The listing builds one solid part. Answer for the finished solid, in the listing's coordinates (mm). Face numbers are marked on the shaded views. A direction names the side the tool comes from. Round coordinates to 2 decimals unless told otherwise and drop trailing zeros. Write each loop counter-clockwise with the first axis right and the second up, starting at its lowest first coordinate (ties: lowest second). Pieces come first, ordered by that corner, then holes. Notation, with made-up numbers: (30, 49) - (85, 49) arc R13 ccw to (85, 54) - close; hole circle Ø11 at (51, -13.75). An arc over 180 degrees is marked (long way). Use a Markdown table: item, result. Add a question column.
1) A tool of negligible diameter and unlimited length cuts with its end or side. For the marked faces 5, 6, 7 and 8, from which of +Z, -Z, +X, -X, +Y, -Y can it reach the whole face along a straight path? Write none if from no direction.
2) A cutting plane is placed at D-D (z = 20.5). Give the vertices of the cut face in (x, y).
3) A cutting plane is placed at B-B (z = 4.5). Give the vertices of the cut face in (x, y), then the cut area to 3 significant figures.
4) Determine the mould class of the marked faces 1, 2, 3 and 4 for opening direction Z: +Z half, -Z half, draft (parallel to the pull), parting line (faces both ways), or undercut.
5) Each of these flat-tipped pins is pushed along its axis until it touches: P1, Ø5, axis at x = 30, z = -11.5, coming from the +Y side; P2, Ø2, axis at x = 35, y = 9, coming from the +Z side; P3, Ø3.5, axis at x = -7, z = 21, coming from the +Y side; P4, Ø5, axis at x = 33, y = 8.5, coming from the -Z side. Where does it stop, or does it pass through?
6) A cutting plane is placed at C-C (x = -27). Give the vertices of the cut face in (y, z), then the cut area to 3 significant figures.
7) A cutting plane is placed at A-A (y = 2). Give the vertices of the cut face in (x, z), then the cut area to 3 significant figures.
8) Find the intervals of material crossed by probe 1 along Z at (x, y) = (-35, 2.1); probe 2 along X at (y, z) = (9.25, -16.5); probe 3 along Z at (x, y) = (4.5, 6.5), in increasing order. Write a range as from..to.
```python
from build123d import *

# Parameters (mm, degrees)
SKETCH_1_W          = 75.5
SKETCH_1_H          = 51.2
EXTRUDE_1_DEPTH     = 4
HOLE_WIZARD_M3_1_D  = 3.2
FILLET_1_R          = 3
SKETCH_4_W          = 9
SKETCH_4_H          = 11
EXTRUDE_2_DEPTH     = 14
CUT_EXTRUDE_1_DEPTH = 12
SKETCH_6_W          = 25
SKETCH_6_H          = 10
EXTRUDE_3_DEPTH     = 10
SKETCH_7_R          = 1.963016799
CUT_EXTRUDE_2_DEPTH = 1
CHAMFER_1_SIZE      = 2
CHAMFER_1_SIZE2     = 3
SKETCH_8_W          = 6.560594773
SKETCH_8_H          = 32.588402295
EXTRUDE_4_DEPTH     = 10
SKETCH_9_W          = 28
SKETCH_9_H          = 18
EXTRUDE_5_DEPTH     = 14.3
SKETCH_10_W         = 28
SKETCH_10_H         = 14.3
SKETCH_10_R         = 1.542197262
CUT_EXTRUDE_3_DEPTH = 5


with BuildPart() as part:
    # 草图1 → 凸台-拉伸1 (new body)
    with BuildSketch(Plane(origin=(0, 0, 0), x_dir=(1, 0, 0), z_dir=(0, 1, 0))):
        Rectangle(SKETCH_1_W, SKETCH_1_H)
    extrude(amount=EXTRUDE_1_DEPTH)

    # M3 间隙孔1 (through all)
    with Locations(Plane(origin=(0, 4, 0), x_dir=(1, 0, 0), z_dir=(0, 1, 0))):
        with Locations((-35, 23), (35, 23), (-35, -23), (35, -23)):
            Hole(HOLE_WIZARD_M3_1_D / 2)

    # 圆角1
    fillet_1_edges = [part.edges().sort_by_distance(p)[0] for p in [
        (-37.75, 2, -25.6),
        (37.75, 2, -25.6),
        (37.75, 2, 25.6),
        (-37.75, 2, 25.6),
    ]]
    fillet(fillet_1_edges, radius=FILLET_1_R)

    # 草图4 → 凸台-拉伸2 (add)
    with BuildSketch(Plane.XY.offset(25.6)):
        with Locations((23.25, 9.5)):
            Rectangle(SKETCH_4_W, SKETCH_4_H)
    extrude(amount=-EXTRUDE_2_DEPTH)

    # 草图5 → 切除-拉伸1 (cut)
    with BuildSketch(Plane(origin=(0, 0, 11.6), x_dir=(-1, 0, 0), z_dir=(0, 0, -1))):
        with BuildLine():
            Line((-27.75, 10.5), (-28.75, 10.5))
            Line((-28.75, 10.5), (-28.75, 16))
            Line((-28.75, 16), (-17.75, 16))
            Line((-17.75, 16), (-17.75, 10.5))
            Line((-17.75, 10.5), (-18.75, 10.5))
            ThreePointArc((-18.75, 10.5), (-23.25, 15), (-27.75, 10.5))
        make_face()
    extrude(amount=-CUT_EXTRUDE_1_DEPTH, mode=Mode.SUBTRACT)

    # 草图6 → 凸台-拉伸3 (add)
    with BuildSketch(Plane(origin=(0, 4, 0), x_dir=(1, 0, 0), z_dir=(0, 1, 0))):
        with Locations((-5.75, -20.6)):
            Rectangle(SKETCH_6_W, SKETCH_6_H)
    extrude(amount=EXTRUDE_3_DEPTH)

    # 草图7 → 切除-拉伸2 (cut)
    with BuildSketch(Plane(origin=(0, 14, 0), x_dir=(1, 0, 0), z_dir=(0, 1, 0))):
        with Locations(Location((-15.05979197, -21.684454558, 0), (0, 0, 270))):
            Circle(SKETCH_7_R)
        with Locations(Location((-8.94020803, -21.684454558, 0), (0, 0, 90))):
            Circle(SKETCH_7_R)
        with Locations(Location((3.55979197, -21.684454558, 0), (0, 0, 90))):
            Circle(SKETCH_7_R)
        with Locations(Location((-2.55979197, -21.684454558, 0), (0, 0, 270))):
            Circle(SKETCH_7_R)
    extrude(amount=-CUT_EXTRUDE_2_DEPTH, mode=Mode.SUBTRACT)

    # 倒角1
    chamfer_1_edges = [part.edges().sort_by_distance(p)[0] for p in [
        (-5.75, 14, 15.6),
    ]]
    chamfer_1_side = [part.faces().sort_by_distance(p)[0] for p in [
        (-5.75, 9, 15.6),
    ]]
    chamfer(chamfer_1_edges, length=CHAMFER_1_SIZE, length2=CHAMFER_1_SIZE2, reference=chamfer_1_side[0])

    # 草图8 → 凸台-拉伸4 (add)
    with BuildSketch(Plane(origin=(0, 4, 0), x_dir=(1, 0, 0), z_dir=(0, 1, 0))):
        with Locations((34.469702614, -0.78179248)):
            Rectangle(SKETCH_8_W, SKETCH_8_H)
    extrude(amount=EXTRUDE_4_DEPTH)

    # 草图9 → 凸台-拉伸5 (add)
    with BuildSketch(Plane(origin=(0, 4, 0), x_dir=(1, 0, 0), z_dir=(0, 1, 0))):
        with Locations((-15.25, 22.6)):
            Rectangle(SKETCH_9_W, SKETCH_9_H)
        with Locations((15.25, 22.6)):
            Rectangle(SKETCH_9_W, SKETCH_9_H)
    extrude(amount=EXTRUDE_5_DEPTH)

    # 草图10 → 切除-拉伸3 (cut)
    # profile 1 of 2: a face of its own
    with BuildSketch(Plane(origin=(0, 0, -31.6), x_dir=(-1, 0, 0), z_dir=(0, 0, -1))):
        with Locations((-15.25, 11.15)):
            Rectangle(SKETCH_10_W, SKETCH_10_H)
        with Locations((-26.769914648, 11.409080509)):
            Circle(SKETCH_10_R, mode=Mode.SUBTRACT)
        with Locations((-3.730085352, 11.409080509)):
            Circle(SKETCH_10_R, mode=Mode.SUBTRACT)
        Polygon((-22.404607637, 8.177619476), (-8.095392363, 8.177619476), (-6.020301502, 15.325154661), (-24.479698498, 15.325154661), align=None, mode=Mode.SUBTRACT)
    # profile 2 of 2: a face of its own
    with BuildSketch(Plane(origin=(0, 0, -31.6), x_dir=(-1, 0, 0), z_dir=(0, 0, -1))):
        with Locations((15.25, 11.15)):
            Rectangle(SKETCH_10_W, SKETCH_10_H)
        with Locations((3.730085352, 11.409080509)):
            Circle(SKETCH_10_R, mode=Mode.SUBTRACT)
        with Locations((26.769914648, 11.409080509)):
            Circle(SKETCH_10_R, mode=Mode.SUBTRACT)
        Polygon((6.020301502, 15.325154661), (8.095392363, 8.177619476), (22.404607637, 8.177619476), (24.479698498, 15.325154661), align=None, mode=Mode.SUBTRACT)
    extrude(amount=-CUT_EXTRUDE_3_DEPTH, mode=Mode.SUBTRACT)


solid = part.part
```
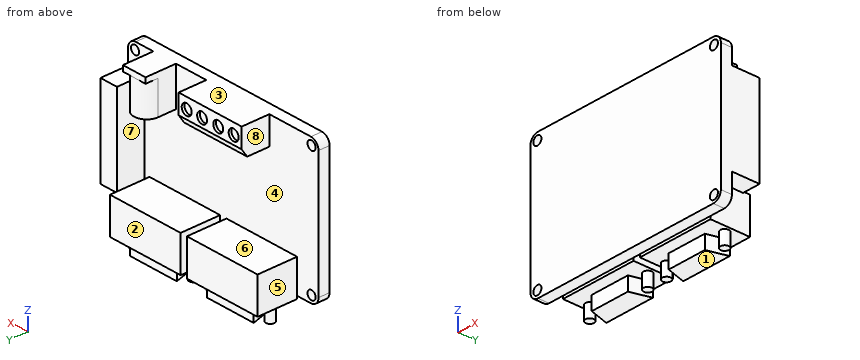
Entries:
| question | item | result |
|---|---|---|
| 1 | face 5 | +Z, -Z, -X, +Y |
| 1 | face 6 | -X, +Y |
| 1 | face 7 | +Z, -Z, +Y |
| 1 | face 8 | +Z, -X, +Y |
| 2 | outline | (-37.75, 0) - (37.75, 0) - (37.75, 4) - (27.75, 4) - (27.75, 10.5) arc R4.5 ccw to (18.75, 10.5) - (18.75, 4) - (6.75, 4) - (6.75, 14) - (5.13, 14) - (5.13, 13) - (1.99, 13) - (1.99, 14) - (-0.99, 14) - (-0.99, 13) - (-4.13, 13) - (-4.13, 14) - (-7.37, 14) - (-7.37, 13) - (-10.51, 13) - (-10.51, 14) - (-13.49, 14) - (-13.49, 13) - (-16.63, 13) - (-16.63, 14) - (-18.25, 14) - (-18.25, 4) - (-37.75, 4) - close |
| 3 | outline | (-37.75, 0) - (37.75, 0) - (37.75, 14) - (31.19, 14) - (31.19, 4) - (-37.75, 4) - close |
| 3 | area | 368 mm² |
| 4 | face 1 | -Z half |
| 4 | face 2 | draft |
| 4 | face 3 | +Z half |
| 4 | face 4 | undercut |
| 5 | P1 | stops at y = 18.3 |
| 5 | P2 | stops at z = 17.08 |
| 5 | P3 | stops at y = 14 |
| 5 | P4 | stops at z = -15.51 |
| 6 | outline | (0, -25.6) - (4, -25.6) - (4, -26.6) - (9.88, -26.6) - (9.88, -31.6) - (12.93, -31.6) - (12.93, -26.6) - (18.3, -26.6) - (18.3, -13.6) - (4, -13.6) - (4, 25.6) - (0, 25.6) - close |
| 6 | area | 406 mm² |
| 7 | outline | (-37.75, -22.6) arc R3 ccw to (-34.75, -25.6) - (34.75, -25.6) arc R3 ccw to (37.75, -22.6) - (37.75, 22.6) arc R3 ccw to (34.75, 25.6) - (-34.75, 25.6) arc R3 ccw to (-37.75, 22.6) - close; hole circle Ø3.2 at (-35, -23); hole circle Ø3.2 at (-35, 23); hole circle Ø3.2 at (35, -23); hole circle Ø3.2 at (35, 23) |
| 7 | area | 3,830 mm² |
| 8 | probe 1 | z = -25.59..-24.6, -21.4..21.4, 24.6..25.59 |
| 8 | probe 2 | x = -29.25..-1.25, 1.25..29.25 |
| 8 | probe 3 | z = -26.6..-13.6, 15.6..25.6 |
